from build123d import *

# Parameters (mm, degrees)
BOSS_EXTRUDE1_DEPTH            = 63
CUT_EXTRUDE1_DEPTH             = 19
CUT_EXTRUDE2_DEPTH             = 19
CUT_EXTRUDE3_REACH             = 36.08
CUT_EXTRUDE3_DIRECTION_2_DEPTH = 16.92
CUT_EXTRUDE4_REACH             = 77
SKETCH6_W                      = 19
SKETCH6_H                      = 12


with BuildPart() as part:
    # Sketch1 → Boss-Extrude1 (new body)
    with BuildSketch(Plane.XY):
        Polygon((38.418907052, 31.947162427), (-36.581092948, -6.052837573), (-36.581092948, -18.052837573), (38.418907052, -18.052837573), align=None)
        Polygon((-24.581092948, 16.027162427), (-24.581092948, 0.027162427), (6.99785442, 16.027162427), align=None)
    extrude(amount=-BOSS_EXTRUDE1_DEPTH)

    # Sketch2 → Cut-Extrude1 (cut)
    with BuildSketch(Plane.XY):
        Polygon((-24.581092948, 16.027162427), (6.99785442, 16.027162427), (-24.581092948, 0.027162427), align=None)
    extrude(amount=-CUT_EXTRUDE1_DEPTH, mode=Mode.SUBTRACT)

    # Sketch3 → Cut-Extrude2 (cut)
    with BuildSketch(Plane(origin=(0, 0, -63), x_dir=(-1, 0, 0), z_dir=(0, 0, -1))):
        Polygon((-6.99785442, 16.027162427), (24.581092948, 16.027162427), (24.581092948, 0.027162427), align=None)
    extrude(amount=-CUT_EXTRUDE2_DEPTH, mode=Mode.SUBTRACT)

    # Sketch4 → Cut-Extrude3 (cut, up to next)
    with BuildSketch(Plane(origin=(0, 16.027162427, 0), x_dir=(1, 0, 0), z_dir=(0, 1, 0)), mode=Mode.PRIVATE) as cut_extrude3_sk1:
        Polygon((-11.581092948, 15), (7.086929483, 15), (13.418907052, 15), (13.418907052, 0), (-11.581092948, 0), align=None)
    cut_extrude3_tool1 = extrude(cut_extrude3_sk1.sketch, amount=-CUT_EXTRUDE3_REACH, mode=Mode.PRIVATE) & part.part
    add(cut_extrude3_tool1.solids().sort_by_distance((0.918907, 16.027162, -7.5))[0], mode=Mode.SUBTRACT)

    # Sketch4 → Cut-Extrude3 direction 2 (cut)
    with BuildSketch(Plane(origin=(0, 16.027162427, 0), x_dir=(1, 0, 0), z_dir=(0, 1, 0))):
        Polygon((-11.581092948, 15), (7.086929483, 15), (13.418907052, 15), (13.418907052, 0), (-11.581092948, 0), align=None)
    extrude(amount=CUT_EXTRUDE3_DIRECTION_2_DEPTH, mode=Mode.SUBTRACT)

    # Sketch6 → Cut-Extrude4 (cut, up to next)
    with BuildSketch(Plane(origin=(38.418907052, 0, 0), x_dir=(0, 0, -1), z_dir=(1, 0, 0)), mode=Mode.PRIVATE) as cut_extrude4_sk1:
        with Locations((31.5, 25.947162427)):
            Rectangle(SKETCH6_W, SKETCH6_H)
    cut_extrude4_tool1 = extrude(cut_extrude4_sk1.sketch, amount=-CUT_EXTRUDE4_REACH, mode=Mode.PRIVATE) & part.part
    add(cut_extrude4_tool1.solids().sort_by_distance((38.418907, 25.947162, -31.5))[0], mode=Mode.SUBTRACT)


solid = part.part
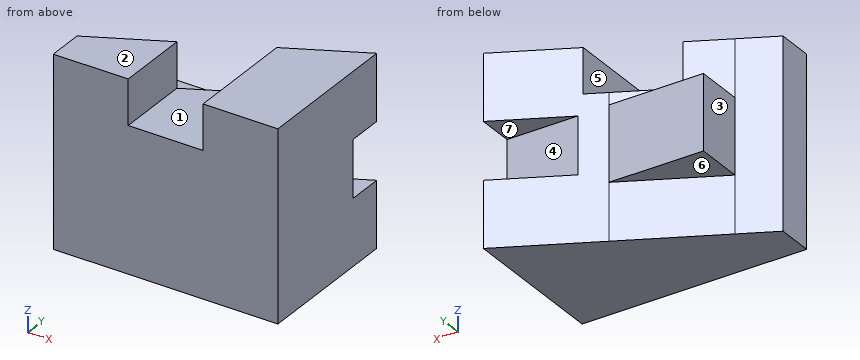
Could you check a few things on this model? Use its own coordinates, in mm. Face numbers are marked on the shaded views. A direction names the side the tool comes from. Round coordinates to 2 decimals unless told otherwise and drop trailing zeros. Order: outer loops, then holes, each group sorted by start corner. A loop starts at its lowest first (then second) coordinate and runs counter-clockwise, first axis right, second up.
Q1. Which directions (+Z, -Z, +X, -X, +Y, -Y) give clear straight access to the entire face, cutting with the end or side of a thin tool? Please do the marked faces 1, 2, 3 and 4.
Geometry says:
face 1: +Z, +Y, -Y
face 2: +Z, +X, -X, +Y, -Y
face 3: +Z, -Z, -X, +Y
face 4: +X, -X, +Y
Q2. I'm going to push flat-ended pins straight in: P1, Ø9.5, axis at x = 21, z = -29, coming from the +Y side; P2, Ø8, axis at y = 5.5, z = -32, coming from the -X side; P3, Ø6, axis at x = -4, y = 20, coming from the -Z side; P4, Ø12, axis at x = 9.5, z = -12, coming from the +Y side. Where does each tip first touch, or does it pass through?
Geometry says:
P1: stops at y = 19.95
P2: stops at x = -24.58
P3: passes through
P4: stops at y = 20.33
Q3. Thinking about a two-plate mould opening in Z: for the marked faces 5, 6 and 7, which applies, released by +Z, released by -Z, zero draft, split by the parting line, or undercut?
Geometry says:
face 5: zero draft
face 6: released by -Z
face 7: undercut
Q4. Please list where these lines run through material, in increasing order: probe 1 along X at (y, z) = (1.5, -25); probe 2 along Y at (x, z) = (5.5, -37); probe 3 along Z at (x, y) = (3, 9).
Geometry says:
probe 1: x = -24.58 to 38.42
probe 2: y = -18.05 to 16.03
probe 3: z = -63 to -15
Q5. Imagine slicing it at A-A, the plane z = -4. List the corners of the cut face in (x, y) for me.
Geometry says:
outline: (-36.58, -18.05) - (-11.58, -18.05) - (-11.58, 6.61) - (-36.58, -6.05) - close; (13.42, -18.05) - (38.42, -18.05) - (38.42, 31.95) - (13.42, 19.28) - close
Q6. Imagine slicing it at C-C, the plane z = -33. List the corners of the cut face in (x, y) for me, then the cut area to 3 significant figures.
Geometry says:
outline: (-36.58, -18.05) - (38.42, -18.05) - (38.42, 19.95) - (14.73, 19.95) - (7, 16.03) - (-24.58, 16.03) - (-24.58, 0.03) - (-36.58, -6.05) - close
area: 2,440 mm2
Q7. Imagine slicing it at B-B, the plane y = -9. List the corners of the cut face in (x, z) for me, then the cut area to 3 significant figures.
Geometry says:
outline: (-36.58, -63) - (38.42, -63) - (38.42, 0) - (13.42, 0) - (13.42, -15) - (-11.58, -15) - (-11.58, 0) - (-36.58, 0) - close
area: 4,350 mm2
Q8. Imagine slicing it at D-D, the plane x = -29.5. List the corners of the cut face in (y, z) for me.
Geometry says:
outline: (-18.05, -63) - (-2.47, -63) - (-2.47, 0) - (-18.05, 0) - close
